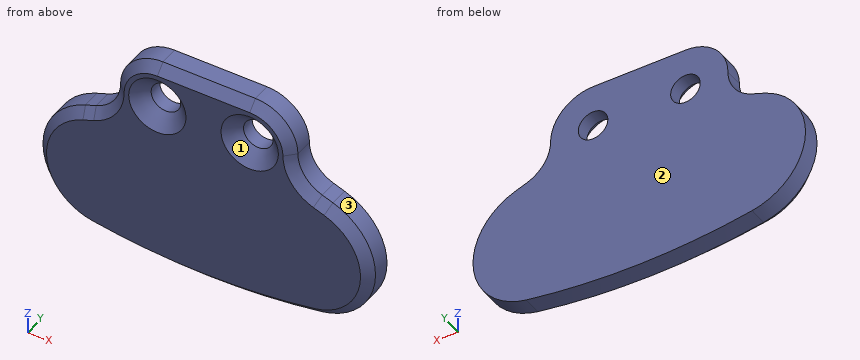
Autodesk Inventor part; units mm, degrees
ref_plane "YZ Plane" through (0, 0, 0) normal (1, 0, 0) x (0, 1, 0)
ref_plane "XZ Plane" through (0, 0, 0) normal (0, 1, 0) x (-1, 0, 0)
ref_plane "XY Plane" through (0, 0, 0) normal (0, 0, 1) x (1, 0, 0)
sketch "Skizze1" plane through (0, 0, 0) normal (0, 1, 0) x (-1, 0, 0)
  circle A0 centre (0, 0) radius 1.6
  circle A1 centre (-10, 0) radius 1.6
  line L0 (0, 4.6) -> (-10, 4.6)
  arc A2 (-10, 4.6) -> (-14.6, 0) centre (-10, 0) ccw
  arc A3 (-17.2319, -3.7588) -> (-14.6, 0) centre (-18.6, 0) ccw
  arc A4 (4.6, 0) -> (0, 4.6) centre (0, 0) ccw
  arc A5 (4.6, 0) -> (7.2319, -3.7588) centre (8.6, 0) ccw
  line L1 (7.2319, -3.7588) -> (8.3941, -4.1818)
  arc A6 (7.2222, -17.6521) -> (8.3941, -4.1818) centre (6, -10.7596) ccw
  arc A7 (-17.2222, -17.6521) -> (7.2222, -17.6521) centre (-5, 51.2726) ccw
  line L2 (-17.2319, -3.7588) -> (-18.3941, -4.1818)
  arc A8 (-18.3941, -4.1818) -> (-17.2222, -17.6521) centre (-16, -10.7596) ccw
  dimension "d0" = 10
  dimension "d1" = 3.2
  dimension "d2" = 3
  dimension "d4" = 4
  dimension "d22" = 7
  dimension "d23" = 20
  dimension "d24" = 22
  dimension "d25" = 70
extrude "Extrusion1" add sketch "Skizze1" along normal blind 3
chamfer "Fase1" distance 1 angle 45 10 edges at (13.2527, 0, 3.2527) (15.3234, 0, -2.2943) (17.813, 0, -3.9703) (22.9737, 0, -11.3663) (5, 0, -18.7274) (-12.9737, 0, -11.3663) (-7.813, 0, -3.9703) (-5.3234, 0, -2.2943) (-3.2527, 0, 3.2527) (5, 0, 4.6)
chamfer "Fase3" distance 1.5 angle 45 2 edges at (11.6, 0, 0) (1.6, 0, 0)
properties part number "_3D-Druck"
Verification items for the finished model (mm, model axes). Face numbers are marked on the shaded views. Coordinates: 2 decimals unless noted, no trailing zeros. Put each result on its own line as item: value. Start each with the question number.
1. Material ranges on L1, parallel to X at y = 0.3, z = 1; L2, parallel to X at y = 0.45, z = 1; L3, parallel to Z at x = 10, y = 2.55, recorded low to high. Write a range as [from, to].
2. Mould release check, pull along Z, two halves, no side actions. Record for the marked faces 1, 2 and 3: released by +Z, released by -Z, zero draft, split by the parting line, or undercut.
3. Go/stop test with flat-tipped pins: pin 1 Ø1.9 at (x, z) = (10, 0) entering from -Y; pin 2 Ø1.5 at (x, y) = (-8.5, 2.5) entering from -Z. Record where each tip stops, or that it passes through.
Computed:
1. L1: [-3.77, -2.62], [2.62, 7.38], [12.62, 13.77]
1. L2: [-3.92, -2.45], [2.45, 7.55], [12.45, 13.92]
1. L3: [-18.55, -1.6], [1.6, 4.6]
2. face 1: undercut
2. face 2: zero draft
2. face 3: split by the parting line
3. pin 1: through
3. pin 2: z = -17.54
